Check sheet for the modelled part. Datum: model origin and axes. Units: mm. A direction names the side the tool comes from. Round coordinates to 2 decimals unless told otherwise and drop trailing zeros.
Item 1: Release check for a two-part mould opening along X. For faces 3 (the flat face through (7, 0, 1)), 4 (the cylindrical face through (3.45, -8.5, -94.22)), 5 (the conical face through (3.34, -6.63, -36.28)) record: pulls with the +X half, pulls with the -X half, needs draft (parallel to the pull), parting line crosses it, or undercut.
Item 2: Set-up check for faces 1 (the flat face through (0, 0, 1)), 2 (the cylindrical face through (4, -9.8, 37.9)): record each of +Z, -Z, +X, -X, +Y, -Y from which the full face is reachable in a straight line by a thin tool's end or side.
Item 3: Material ranges on line 1 along Y through (x, z) = (5, -95.65) (3 decimals); line 2 along Z through (x, y) = (1.5, 8.95); line 3 along Z through (x, y) = (3.5, -10.1) (3 decimals), recorded low to high.
Autodesk Inventor part; units mm, degrees
ref_plane "YZ Plane" through (0, 0, 0) normal (1, 0, 0) x (0, 1, 0)
ref_plane "XZ Plane" through (0, 0, 0) normal (0, 1, 0) x (-1, 0, 0)
ref_plane "XY Plane" through (0, 0, 0) normal (0, 0, 1) x (1, 0, 0)
sketch "Sketch1" plane through (0, 0, 0) normal (1, 0, 0) x (0, 1, 0)
  line L0 (-12.375, 99.15) -> (12.375, 99.15)
  line L1 (12.375, 99.15) -> (12.375, -99.15)
  line L2 (12.375, -99.15) -> (-12.375, -99.15)
  line L3 (-12.375, -99.15) -> (-12.375, 99.15)
  line L4 (-12.375, 99.15) -> (12.375, -99.15) construction
  line L5 (12.375, 99.15) -> (-12.375, -99.15) construction
  point P0 (0, 0)
  dimension "d0" = 198.3
  dimension "d1" = 24.75
extrude "Extrusion1" add sketch "Sketch1" along normal blind 7
sketch "Sketch2" plane through (7, 0, 0) normal (1, 0, 0) x (0, 0, -1)
  circle A0 centre (-95.65, 8.95) radius 1.5
  line L0 (-99.15, 12.375) -> (-99.15, -12.375)
  line L1 (99.15, 12.375) -> (-99.15, 12.375)
  line L2 (-113.68, 5.525) -> (-113.68, 12.375)
  point P0 (0, 0)
  dimension "d4" = 3.5
  dimension "d5" = 3.425
  dimension "d13" = 3
hole "Hole1" at (7, 8.95, 95.65) direction (-1, 0, 0) diameter 3 end through all
mirror "Mirror1" about plane through (0, 0, 0) normal (0, 1, 0) of "Hole1"
mirror "Mirror2" about plane through (0, 0, 0) normal (0, 0, 1) of "Hole1", "Mirror1"
sketch "Sketch3" plane through (0, -12.375, -99.15) normal (0, -1, 0) x (1, 0, 0)
  circle A0 centre (3.5, 62.665) radius 1.5
  line L0 (7, 198.3) -> (7, 0)
  line L1 (0, 0) -> (7, 0)
  point P0 (0, 99.15)
  point P1 (3.5, 0)
  dimension "d14" = 3
  dimension "d15" = 3.5
  dimension "d16" = 62.665
hole "Hole2" at (3.5, -12.375, -36.485) direction (0, 1, 0) diameter 3 depth 5 tip angle 118
mirror "Mirror3" about plane through (0, 0, 0) normal (0, 0, 1) of "Hole2"
properties part number "Mold_sideWall"
Values found:
1. face 3: pulls with the +X half
1. face 4: needs draft
1. face 5: undercut
2. face 1: +Z, -Z, -X, +Y, -Y
2. face 2: -Y
3. line 1: y = -12.375 to -10.45, -7.45 to 7.45, 10.45 to 12.375
3. line 2: z = -99.15 to -97.15, -94.15 to 94.15, 97.15 to 99.15
3. line 3: z = -99.15 to -96.613, -94.687 to -37.985, -34.985 to 34.985, 37.985 to 94.687, 96.613 to 99.15
